Geometry check sheet. Reference: drawing and pictorial views, mm from the part's lowest x, y, z. Round coordinates to 2 decimals unless told otherwise and drop trailing zeros. Loops run counter-clockwise (first coordinate to the right, second up) from the corner with the lowest first, then second, coordinate; pieces in that order, holes last. Notation, with made-up numbers: M 73.25,5 L 80.25,5 A19 cw 80.25,27 Z; hole C 59.5,-24.75 d6. An arc over 180 degrees is marked long. One line per question, with ' | ' between items. Start each with the question number.
(1) Thickness scan on probe 1 along X at (y, z) = (1.9, 23.4); probe 2 along Z at (x, y) = (23.6, 1.1). Record the ranges inside material, lowest first. Write a range as [from, to].
(2) Section check B-B (y = 1.65). Record the boundary of the cut face in (x, z), and give its area (3 significant figures).
(3) Section check A-A (x = 3.4). Record the boundary of the cut face in (y, z), and give its area (3 significant figures).
(4) Section check C-C (z = 3.2). Record the boundary of the cut face in (x, y).
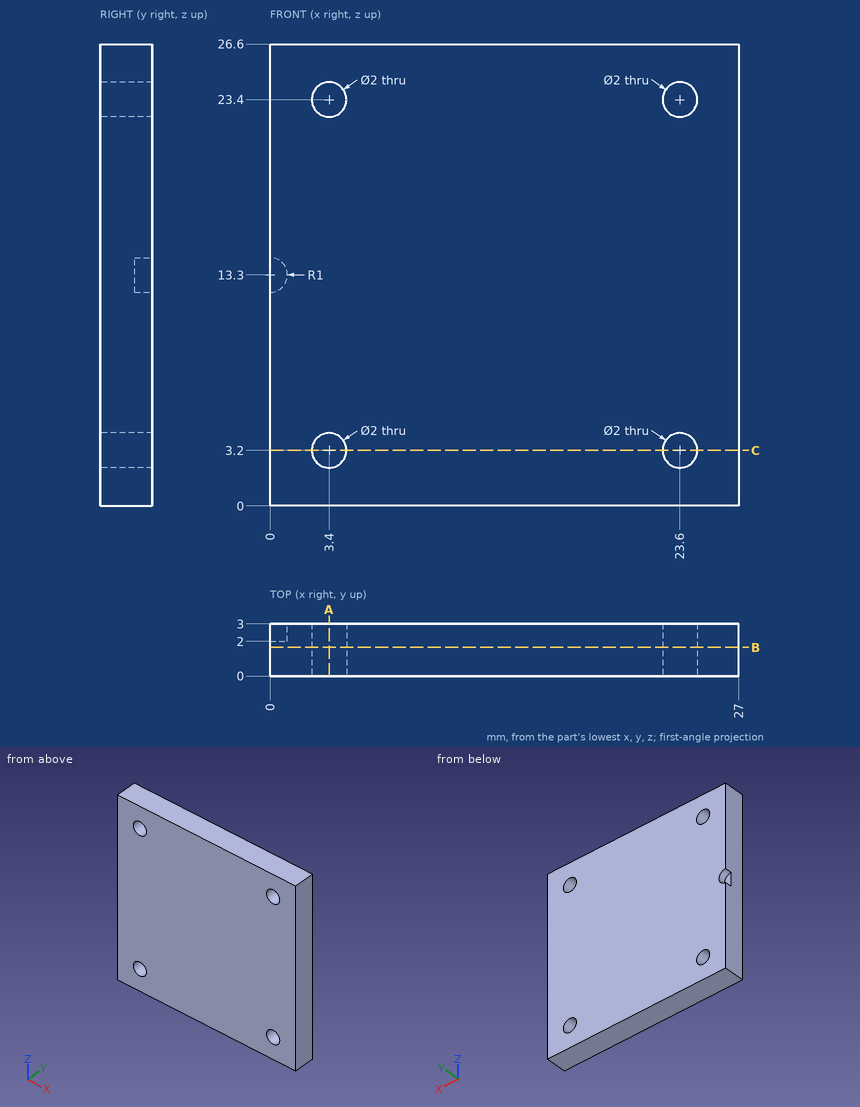
The answers:
1) probe 1: [0, 2.4], [4.4, 22.6], [24.6, 27] | probe 2: [0, 2.2], [4.2, 22.4], [24.4, 26.6]
2) outline: M 0,0 L 27,0 L 27,26.6 L 0,26.6 Z; hole C 3.4,3.2 d2; hole C 3.4,23.4 d2; hole C 23.6,3.2 d2; hole C 23.6,23.4 d2 | area: 706 mm²
3) outline: M 0,0 L 3,0 L 3,2.2 L 0,2.2 Z; M 0,4.2 L 3,4.2 L 3,22.4 L 0,22.4 Z; M 0,24.4 L 3,24.4 L 3,26.6 L 0,26.6 Z | area: 67.8 mm²
4) outline: M 0,0 L 2.4,0 L 2.4,3 L 0,3 Z; M 4.4,0 L 22.6,0 L 22.6,3 L 4.4,3 Z; M 24.6,0 L 27,0 L 27,3 L 24.6,3 Z
